Input: part model. Units: mm. Frame: model coordinates. A direction names the side the tool comes from. Round coordinates to 2 decimals unless told otherwise and drop trailing zeros. Loops run counter-clockwise (first coordinate to the right, second up) from the corner with the lowest first, then second, coordinate; pieces in that order, holes last. Notation, with made-up numbers: (88, -38.5) - (124, -38.5) arc R27 ccw to (124, -12.5) - close; hole circle Ø11 at (9.5, -35). An arc over 180 degrees is marked (long way). Use CSV: the item, a comma, the result in double quotes. Start each with the question number.
1. Access query for faces 1 (the flat face through (17, -10, 3)), 2 (the flat face through (0, -22.5, 9)), 3 (the flat face through (-15.7, -8.81, 8.92)), 4 (the flat face through (21.324, 13.137, 8.874)), 5 (the flat face through (11, 7, 3)). Directions: +Z, -Z, +X, -X, +Y, -Y. A direction counts if a zero-diameter tool reaches every point of the face in a straight line with its end or side. Return the directions, or none.
2. Material intervals for probe 1 along Y at (x, z) = (0, 9); probe 2 along Z at (x, y) = (-11, 9); probe 3 along X at (y, z) = (-23.5, 6), sorted ascending. Write a range as from..to.
3. Cut plane C-C (x = -9). Return loops of the section in (y, z).
4. Cut plane B-B (y = 0). Return loops of the section in (x, z).
5. Cut plane D-D (z = 16). Return loops of the section in (x, y), and give its area (3 significant figures).
6. Pin query (flat end, axial travel): P1, Ø1.5, axis at y = -25.5, z = 12.5, coming from the -X side; P2, Ø8, axis at x = 0.5, y = 6, coming from the -Z side; P3, Ø1, axis at x = 8, z = 2.5, coming from the +Y side; P4, Ø5.5, axis at y = -25.5, z = 5.5, coming from the +X side. Return the tip coordinate at first contact, or that it passes through.
7. Pull-direction query (X, two-part tool) for faces 6 (the cylindrical face through (-6.691, -12.864, 8.916)), 7 (the flat face through (15.48, -9.19, 8.92)), 8 (the flat face through (-10, 8, 18)); classes: +X half, -X half, draft (parallel to the pull), parting line (faces both ways), or undercut.
8. Cut plane A-A (z = 13.5). Return loops of the section in (x, y).
```python
from build123d import *

# Parameters (mm, degrees)
BASE_EXTRUDE_DEPTH           = 18
COMBUSTION_CHAMBER_PROFILE_R = 14.5
CUT_EXTRUDE1_DEPTH           = 12
SKETCH6_R                    = 12.5
CUT_EXTRUDE5_DEPTH           = 19


with BuildPart() as part:
    # rotor profile → Base-Extrude (new body)
    with BuildSketch(Plane.XY):
        with BuildLine():
            Line((-24.173095266, 13.130970823), (-22.181236837, 11.980970823))
            Line((-22.181236837, 11.980970823), (-19.842968247, 10.630970823))
            Line((-19.842968247, 10.630970823), (-19.485571583, 11.250000003))
            Line((-19.485571583, 11.250000003), (-19.128174923, 11.869029177))
            Line((-19.128174923, 11.869029177), (-21.466443514, 13.219029177))
            Line((-21.466443514, 13.219029177), (-23.458301942, 14.369029177))
            ThreePointArc((-23.458301942, 14.369029177), (-12.161921268, 19.163134144), (0, 20.8))
            ThreePointArc((0, 20.8), (12.161921268, 19.163134144), (23.458301942, 14.369029177))
            Line((23.458301942, 14.369029177), (19.128174923, 11.869029177))
            Line((19.128174923, 11.869029177), (19.485571585, 11.25))
            Line((19.485571585, 11.25), (19.842968247, 10.630970823))
            Line((19.842968247, 10.630970823), (24.173095266, 13.130970823))
            ThreePointArc((24.173095266, 13.130970823), (22.676721619, 0.950965705), (18.013328399, -10.4))
            ThreePointArc((18.013328399, -10.4), (10.514800351, -20.114099849), (0.714793324, -27.5))
            Line((0.714793324, -27.5), (0.714793324, -22.5))
            Line((0.714793324, -22.5), (0, -22.5))
            Line((0, -22.5), (-0.714793324, -22.5))
            Line((-0.714793324, -22.5), (-0.714793324, -27.5))
            ThreePointArc((-0.714793324, -27.5), (-10.514800351, -20.114099849), (-18.013328399, -10.4))
            ThreePointArc((-18.013328399, -10.4), (-22.676721619, 0.950965705), (-24.173095266, 13.130970823))
        make_face()
    extrude(amount=BASE_EXTRUDE_DEPTH)

    # combustion chamber profile → Cut-Extrude1 (cut)
    with BuildSketch(Plane(origin=(0, 0, 3), x_dir=(-1, 0, 0), z_dir=(0, 0, -1))):
        Circle(COMBUSTION_CHAMBER_PROFILE_R)
        Polygon((18, 21), (18, 18), (0, 18), (-18, 18), (-18, 21), align=None)
        Polygon((-9.186533479, -26.088457268), (-27.186533479, 5.088457268), (-24.588457268, 6.588457268), (-15.588457268, -9), (-6.588457268, -24.588457268), align=None)
        Polygon((27.186533479, 5.088457268), (9.186533479, -26.088457268), (6.588457268, -24.588457268), (15.588457268, -9), (24.588457268, 6.588457268), align=None)
    extrude(amount=-CUT_EXTRUDE1_DEPTH, mode=Mode.SUBTRACT)

    # Sketch6 → Cut-Extrude5 (cut, through all)
    with BuildSketch(Plane(origin=(0, 0, 18), x_dir=(-1, 0, 0), z_dir=(0, 0, -1))):
        Circle(SKETCH6_R)
    extrude(amount=CUT_EXTRUDE5_DEPTH, mode=Mode.SUBTRACT)


solid = part.part
```
Established:
1,face 1,"+X, -Y"
1,face 2,"+Z, -Z, -Y"
1,face 3,"-X, -Y"
1,face 4,"+Z, -Z"
1,face 5,"none"
2,probe 1,"y = -22.5..-14.5, 14.5..18"
2,probe 2,"z = 0..3, 15..18"
2,probe 3,"x = -6.69..-0.71, 0.71..6.69"
3,outline,"(-21.55, 0) - (-8.67, 0) - (-8.67, 3) - (-11.37, 3) - (-11.37, 15) - (-8.67, 15) - (-8.67, 18) - (-21.55, 18) - (-21.55, 15) - (-20.41, 15) - (-20.41, 3) - (-21.55, 3) - close; (8.67, 0) - (19.91, 0) - (19.91, 3) - (18, 3) - (18, 15) - (19.91, 15) - (19.91, 18) - (8.67, 18) - (8.67, 15) - (11.37, 15) - (11.37, 3) - (8.67, 3) - close"
4,outline,"(-22.42, 0) - (-12.5, 0) - (-12.5, 3) - (-14.5, 3) - (-14.5, 15) - (-12.5, 15) - (-12.5, 18) - (-22.42, 18) - (-22.42, 15) - (-20.78, 15) - (-20.78, 3) - (-22.42, 3) - close; (12.5, 0) - (22.42, 0) - (22.42, 3) - (20.78, 3) - (20.78, 15) - (22.42, 15) - (22.42, 18) - (12.5, 18) - (12.5, 15) - (14.5, 15) - (14.5, 3) - (12.5, 3) - close"
5,outline,"(-24.17, 13.13) arc R46 ccw to (-0.71, -27.5) - (-0.71, -22.5) - (0.71, -22.5) - (0.71, -27.5) arc R46 ccw to (24.17, 13.13) - (19.84, 10.63) - (19.13, 11.87) - (23.46, 14.37) arc R46 ccw to (-23.46, 14.37) - (-19.13, 11.87) - (-19.84, 10.63) - close; hole circle Ø25 at (0, 0)"
5,area,"1,170 mm2"
6,P1,"stops at x = -5.03"
6,P2,"passes through"
6,P3,"stops at y = 20.18"
6,P4,"stops at x = 7.61"
7,face 6,"undercut"
7,face 7,"+X half"
7,face 8,"draft"
8,outline,"(-24.17, 13.13) arc R46 ccw to (-23.49, 4.69) - (-7.69, -22.69) arc R46 ccw to (-0.71, -27.5) - (-0.71, -22.5) - (0.71, -22.5) - (0.71, -27.5) arc R46 ccw to (7.69, -22.69) - (23.49, 4.69) arc R46 ccw to (24.17, 13.13) - (19.84, 10.63) - (19.13, 11.87) - (23.46, 14.37) arc R46 ccw to (15.8, 18) - (-15.8, 18) arc R46 ccw to (-23.46, 14.37) - (-19.13, 11.87) - (-19.84, 10.63) - close; hole circle Ø29 at (0, 0)"
